Input: dimensioned drawing with shaded views. Units: mm. Origin: part minimum x, y, z. Coordinates: 2 decimals unless noted, no trailing zeros. Order: outer loops, then holes, each group sorted by start corner. A loop starts at its lowest first (then second) coordinate and runs counter-clockwise, first axis right, second up. Notation, with made-up numbers: M -33.75,30.25 L 15.25,30.25 A23 ccw 15.25,49.25 Z; hole C 17.5,-40 d8. An arc over 180 degrees is marked long. Use CSV: the item, a comma, the result in double quotes. Start each with the question number.
1. Pull-direction query (X, two-part tool) for the marked faces 1, 2, 3 and 4; classes: pulls with the +X half, pulls with the -X half, needs draft (parallel to the pull), parting line crosses it, or undercut.
2. Section query C-C on z = 19.5. Return the cut outline in (x, y) (1 decimal).
3. Section query B-B on x = 9.5. Return the cut outline in (y, z) (1 decimal).
4. Section query A-A on y = 4.5. Return the cut outline in (x, z).
5. Material intervals for line 1 (X direction, y = 7.75, z = 6.5) (1 decimal); line 2 (X direction, y = 1, z = 6) (1 decimal); line 3 (X direction, y = 1.25, z = 15.5) (1 decimal), sorted ascending.
6. Section query D-D on x = 32.5. Return the cut outline in (y, z) (1 decimal), and give its area (3 significant figures).
7. First-contact query: P1, Ø6.5, axis at x = 60, z = 36.83, coming from the +Y side (3 decimals); P2, Ø1, axis at x = 34, y = 1, coming from the +Z side (1 decimal); P3, Ø3, axis at x = 31, y = 6.5, coming from the +Z side (1 decimal); P4, Ø4, axis at x = 79, y = 6.5, coming from the +Z side. Flat tips, straight axial feed; report the tip coordinate or a pass-through.
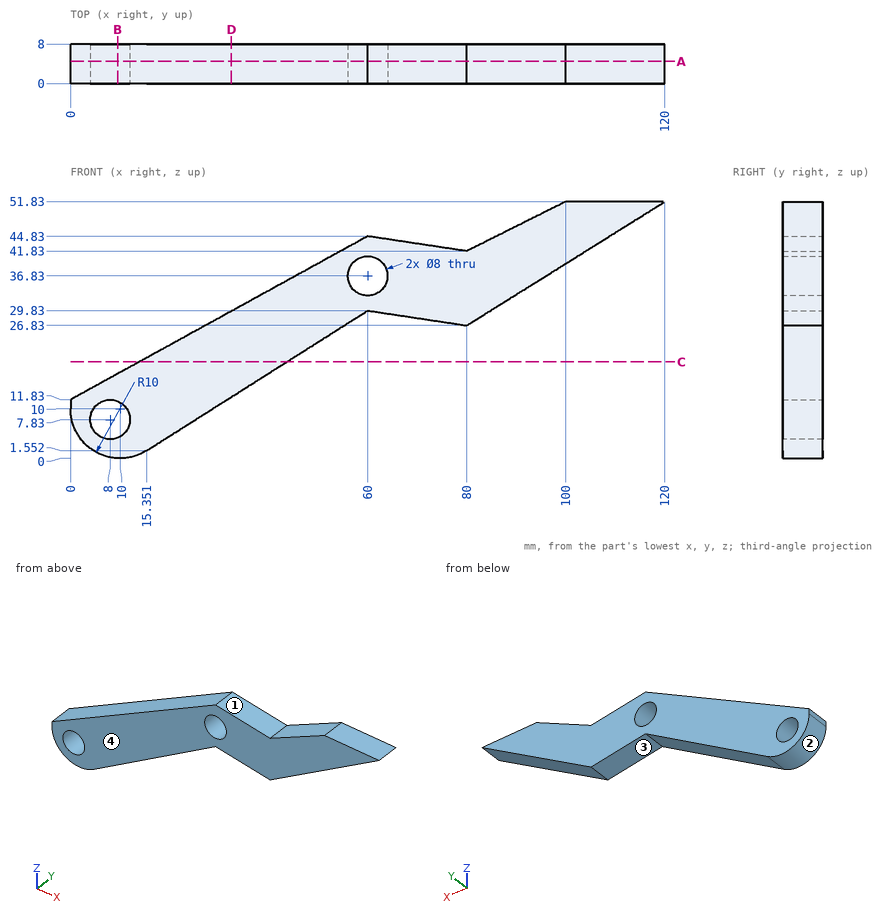
Results list:
1,face 1,"undercut"
1,face 2,"parting line crosses it"
1,face 3,"undercut"
1,face 4,"needs draft"
2,outline,"M 13.9,0 L 43.7,0 L 43.7,8 L 13.9,8 Z"
3,outline,"M 0,0 L 8,0 L 8,4.1 L 0,4.1 Z; M 0,11.5 L 8,11.5 L 8,17.1 L 0,17.1 Z"
4,outline,"M 0,10 A10 ccw 15.35,1.55 L 60,29.83 L 80,26.83 L 120,51.83 L 100,51.83 L 80,41.83 L 60,44.83 L 0,11.83 Z; hole C 8,7.83 d8; hole C 60,36.83 d8"
5,line 1,"x = 0.6 to 4.2, 11.8 to 23.2"
5,line 2,"x = 0.8 to 4.4, 11.6 to 22.4"
5,line 3,"x = 6.7 to 37.4"
6,outline,"M 0,12.4 L 8,12.4 L 8,29.7 L 0,29.7 Z"
6,area,"138 mm²"
7,P1,"passes through"
7,P2,"stops at z = 30.8"
7,P3,"stops at z = 29.7"
7,P4,"stops at z = 42.33"
